Input: part model. Units: mm. Frame: model coordinates. Round coordinates to 2 decimals unless told otherwise and drop trailing zeros. Order: outer loops, then holes, each group sorted by start corner. A loop starts at its lowest first (then second) coordinate and runs counter-clockwise, first axis right, second up. Notation, with made-up numbers: (5.5, -31) -> (43.5, -31) arc R26 cw to (43.5, 0) -> close; hole circle Ø1 at (41.25, -11). An arc over 180 degrees is marked (long way). Answer as CSV lines item,"result". Start each with the question number.
1) First-contact query: P1, Ø5, axis at y = -18, z = 17, coming from the +X side; P2, Ø4, axis at x = -15.5, z = 33.5, coming from the -Y side; P3, Ø1.5, axis at x = -2.5, z = 4, coming from the +Y side. Flat tips, straight axial feed; report the tip coordinate or a pass-through.
2) Line query: L1, parallel to Y at x = 1, z = 2; L2, parallel to Y at x = 1, z = 26; L3, parallel to Z at x = 4.5, y = 23. Output: solid intervals per line, ascending.
3) Section query C-C, the plane z = 35.5. Output: boundary loops of the cut face in (x, y).
4) Section query B-B, the plane x = 12. Output: boundary loops of the cut face in (y, z), and give its area (3 significant figures).
5) Mould query, pull axis Y, two halves, no side actions, for faces 1 (the face through (-2.996, 14.887, 1.479)), 2 (the face through (-24.19, 0, 1)), 3 (the face through (31.29, 1.08, 1.48)). Classes: +Y half, -Y half, draft (parallel to the pull), parting line (faces both ways), or undercut.
6) Section query D-D, the plane x = -7.5. Output: boundary loops of the cut face in (y, z), and give its area (3 significant figures).
7) Section query A-A, the plane y = 0. Output: boundary loops of the cut face in (x, z).
Autodesk Inventor part; units mm, degrees
ref_plane "YZ Plane" through (0, 0, 0) normal (1, 0, 0) x (0, 1, 0)
ref_plane "XZ Plane" through (0, 0, 0) normal (0, 1, 0) x (-1, 0, 0)
ref_plane "XY Plane" through (0, 0, 0) normal (0, 0, 1) x (1, 0, 0)
ref_plane "Work Plane1" through (0, 0, 0) normal (0, 0, 1) x (1, 0, 0)
sketch "Sketch1" plane through (0, 0, 0) normal (0, 0, 1) x (1, 0, 0)
  circle A0 centre (27.1062, 0) radius 1.75 construction
  circle A1 centre (-19.5414, -18) radius 1.75 construction
  circle A2 centre (-19.5414, 18) radius 1.75 construction
  arc A3 (-24.1905, -18.9934) -> (-24.1905, 18.9934) centre (0.3095, 0) ccw
  circle A4 centre (0.3095, 0) radius 15.25
  circle A5 centre (-19.5414, 18) radius 1.75
  circle A6 centre (-19.5414, -18) radius 1.75
  circle A7 centre (27.1062, 0) radius 1.75
  line L0 (-24.1905, 18.9934) -> (-24.1905, -18.9934)
  arc A8 (-24.1905, -18.9934) -> (-24.1905, 18.9934) centre (0.3095, 0) ccw
  circle A9 centre (0.3095, 0) radius 15.25
  point P0 (0, 0)
extrude "Extrusion1" add sketch "Sketch1" along normal blind 3
sketch "Sketch2" plane through (0, 0, 3) normal (0, 0, 1) x (1, 0, 0)
  circle A0 centre (0.3095, 0) radius 15.25
  circle A1 centre (0.3095, 0) radius 15.3
  circle A2 centre (0.3095, 0) radius 18.3
  point P0 (0, 0)
  dimension "d2" = 30.6
  dimension "d3" = 3
extrude "Extrusion2" add sketch "Sketch2" along normal blind 35 contours A2
properties part number "10_Zeiss_Axiotech_Eypiecemount_Adapter"
Findings:
1,P1,"stops at x = 10.04"
1,P2,"stops at y = -12.01"
1,P3,"stops at y = 18.18"
2,L1,"y = -30.99 to -15.23, 15.23 to 30.99"
2,L2,"y = -18.29 to -15.28, 15.28 to 18.29"
2,L3,"z = 0 to 3"
3,outline,"circle Ø36.6 at (0.31, 0); hole circle Ø30.6 at (0.31, 0)"
4,outline,"(-28.71, 0) -> (-9.79, 0) -> (-9.79, 3) -> (-9.87, 3) -> (-9.87, 38) -> (-14.08, 38) -> (-14.08, 3) -> (-28.71, 3) -> close; (9.79, 0) -> (28.71, 0) -> (28.71, 3) -> (14.08, 3) -> (14.08, 38) -> (9.87, 38) -> (9.87, 3) -> (9.79, 3) -> close"
4,area,"408 mm^2"
5,face 1,"undercut"
5,face 2,"draft"
5,face 3,"parting line"
6,outline,"(-30, 0) -> (-13.1, 0) -> (-13.1, 3) -> (-13.16, 3) -> (-13.16, 38) -> (-16.55, 38) -> (-16.55, 3) -> (-30, 3) -> close; (13.1, 0) -> (30, 0) -> (30, 3) -> (16.55, 3) -> (16.55, 38) -> (13.16, 38) -> (13.16, 3) -> (13.1, 3) -> close"
6,area,"339 mm^2"
7,outline,"(-24.19, 0) -> (-14.94, 0) -> (-14.94, 3) -> (-14.99, 3) -> (-14.99, 38) -> (-17.99, 38) -> (-17.99, 3) -> (-24.19, 3) -> close; (15.56, 0) -> (25.36, 0) -> (25.36, 3) -> (18.61, 3) -> (18.61, 38) -> (15.61, 38) -> (15.61, 3) -> (15.56, 3) -> close; (28.86, 0) -> (31.31, 0) -> (31.31, 3) -> (28.86, 3) -> close"
